Design review of the part built by this model. Coordinates are the model's own, in mm. A direction names the side the tool comes from. Give positions to 0.01 mm unless a question says otherwise; leave off trailing zeros. Write each loop counter-clockwise with the first axis right and the second up, starting at its lowest first coordinate (ties: lowest second). Pieces come first, ordered by that corner, then holes.
```python
from build123d import *

# Parameters (mm, degrees)
BOSS_EXTRUDE1_DEPTH = 10
BOSS_EXTRUDE5_DEPTH = 15


with BuildPart() as part:
    # Sketch1 → Boss-Extrude1 (new body)
    with BuildSketch(Plane.XY):
        with BuildLine():
            Line((0, 20), (0, 0))
            Line((0, 0), (30, 0))
            ThreePointArc((30, 0), (18.027756377, 14.541634566), (0, 20))
        make_face()
    extrude(amount=BOSS_EXTRUDE1_DEPTH)

    # Sketch2 → Boss-Extrude5 (add)
    with BuildSketch(Plane.XY.offset(10)):
        with BuildLine():
            Line((0, 5), (0, 0))
            Line((0, 0), (30, 0))
            Line((30, 0), (30, 25))
            ThreePointArc((30, 25), (21.654721001, 22.464201476), (16.131034824, 15.71417579))
            ThreePointArc((16.131034824, 15.71417579), (10.026103583, 7.405271123), (0, 5))
        make_face()
    extrude(amount=BOSS_EXTRUDE5_DEPTH)


solid = part.part
```
(1) To check wall thickness, follow L1, parallel to Z at x = 4, y = 10.75; L2, parallel to Z at x = 26, y = 17; L3, parallel to Y at x = 8.5, z = 18. State the ranges of each line that lie inside material, in increasing order.
Resolved:
L1: z = 0 to 10
L2: z = 10 to 25
L3: y = 0 to 6.52
(2) Consider section C-C, the plane y = 7.5. Give the boundary of the cut face in (x, z).
Resolved:
outline: (0, 0) - (25.62, 0) - (25.62, 10) - (30, 10) - (30, 25) - (10.17, 25) - (10.17, 10) - (0, 10) - close
(3) Consider section D-D, the plane x = 5.25. Give the boundary of the cut face in (y, z).
Resolved:
outline: (0, 0) - (19.57, 0) - (19.57, 10) - (5.32, 10) - (5.32, 25) - (0, 25) - close
(4) Clearance check with flat-ended pins moving along their axes: P1, Ø7.5, axis at x = 6.5, y = 10.5, coming from the +Z side; P2, Ø4, axis at y = 3.5, z = 4.5, coming from the +X side; P3, Ø4, axis at y = 8, z = 5.5, coming from the +X side. State where each tip first meets the part, or that it passes through.
Resolved:
P1: stops at z = 10
P2: stops at x = 29.33
P3: stops at x = 26.72
(5) Consider section A-A, the plane y = 16.5. Give the boundary of the cut face in (x, z), then the cut area to 3 significant figures.
Resolved:
outline: (0, 0) - (14.67, 0) - (14.67, 10) - (0, 10) - close; (16.48, 10) - (30, 10) - (30, 25) - (16.48, 25) - close
area: 349 mm2
(6) Consider section B-B, the plane z = 5.5. Give the boundary of the cut face in (x, y), then the cut area to 3 significant figures.
Resolved:
outline: (0, 0) - (30, 0) arc R32.5 ccw to (0, 20) - close
area: 434 mm2
(7) Tool access review of faces 1 (the face through (18, 10, 25)), 2 (the face through (6, 13, 10)), 3 (the face through (18.25, 14.39, 4.93)): name each direction out of +Z, -Z, +X, -X, +Y, -Y from which nothing blocks a thin tool from reaching the whole face with its end or side.
Resolved:
face 1: +Z, +X, -X, +Y, -Y
face 2: +Z, -X, +Y
face 3: -Z, +X, +Y
